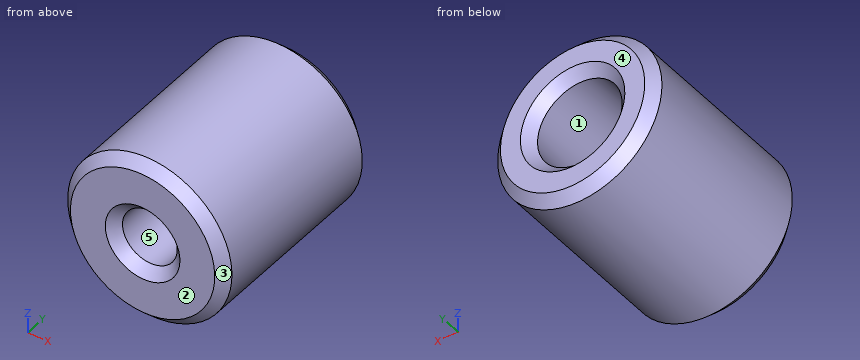
```python
from build123d import *

# Parameters (mm, degrees)
CHAMFER1_SIZE = 1


with BuildPart() as part:
    # Sketch1 → Revolve1 (revolve)
    with BuildSketch(Plane(origin=(0, 0, 0), x_dir=(0, 0, -1), z_dir=(1, 0, 0)), mode=Mode.PRIVATE) as revolve1_sk:
        Polygon((-4.25, 20), (-4.25, 12), (-2.75, 8), (-2.75, 0), (-8.25, 0), (-8.25, 20), align=None)
    revolve(revolve1_sk.sketch.rotate(Axis((0, 0, 0), (0, 1, 0)), 180), axis=Axis((0, 0, 0), (0, 1, 0)))

    # Chamfer1
    chamfer1_edges = [part.edges().sort_by_distance(p)[0] for p in [
        (0, 20, 8.25),
        (0, 0, 8.25),
        (0, 0, 2.75),
        (0, 20, 4.25),
    ]]
    chamfer(chamfer1_edges, length=CHAMFER1_SIZE)


solid = part.part
```
Read the model definition and answer for the solid it produces. Units are mm, in the model's axes. Face numbers are marked on the shaded views. A direction names the side the tool comes from. Give positions to 0.01 mm unless a question says otherwise; leave off trailing zeros. Order: outer loops, then holes, each group sorted by start corner. A loop starts at its lowest first (then second) coordinate and runs counter-clockwise, first axis right, second up. Notation, with made-up numbers: (-15, 55) -> (26, 55) arc R24 ccw to (26, 74) -> close; hole circle Ø8 at (41, 26). An arc over 180 degrees is marked (long way). Write item = value, one per line.
1. A cutting plane is placed at C-C, the plane y = 14.25. Write down the section's boundary in (x, z).
Numbers:
outline = circle Ø16.5 at (0, 0); hole circle Ø8.5 at (0, 0)
2. The mould has two halves that part along Y. Classify the marked faces 3, 4 and 5: +Y half, -Y half, draft (parallel to the pull), parting line (faces both ways), or undercut.
Numbers:
face_3 = -Y half
face_4 = +Y half
face_5 = draft
3. Straight lines are drawn through the part: line 1 along X through (y, z) = (17.75, 0); line 2 along X through (y, z) = (3.25, 0); line 3 along Z through (x, y) = (-1.5, 2.5). For each, find the intervals that lie inside material, in ascending order.
Numbers:
line_1 = -8.25 to -4.25, 4.25 to 8.25
line_2 = -8.25 to -2.75, 2.75 to 8.25
line_3 = -8.11 to -2.3, 2.3 to 8.11
4. For the marked faces 1 and 2, determine the directions among +Z, -Z, +X, -X, +Y, -Y from which every point of the face is accessible in a straight line to the end or side of a thin tool.
Numbers:
face_1 = +Y
face_2 = +Z, -Z, +X, -X, -Y
5. Given pin 1 (1.5 mm diameter, centred on x = -5, z = -6.5, fed in from +Y); pin 2 (9 mm diameter, centred on x = 0, z = 0, fed in from +Y), each flat-ended and moving along its own axis, determine where each tip first touches the part or whether it passes through.
Numbers:
pin_1 = 19.8
pin_2 = 19.25
6. A cutting plane is placed at B-B, the plane x = 0. Write down the section's boundary in (y, z), and give its area (3 significant figures).
Numbers:
outline = (0, -7.25) -> (1, -8.25) -> (19, -8.25) -> (20, -7.25) -> (20, -5.25) -> (19, -4.25) -> (12, -4.25) -> (8, -2.75) -> (1, -2.75) -> (0, -3.75) -> close; (0, 3.75) -> (1, 2.75) -> (8, 2.75) -> (12, 4.25) -> (19, 4.25) -> (20, 5.25) -> (20, 7.25) -> (19, 8.25) -> (1, 8.25) -> (0, 7.25) -> close
area = 186 mm²
7. A cutting plane is placed at A-A, the plane z = 0. Write down the section's boundary in (x, y), and give its area (3 significant figures).
Numbers:
outline = (-8.25, 1) -> (-7.25, 0) -> (-3.75, 0) -> (-2.75, 1) -> (-2.75, 8) -> (-4.25, 12) -> (-4.25, 19) -> (-5.25, 20) -> (-7.25, 20) -> (-8.25, 19) -> close; (2.75, 1) -> (3.75, 0) -> (7.25, 0) -> (8.25, 1) -> (8.25, 19) -> (7.25, 20) -> (5.25, 20) -> (4.25, 19) -> (4.25, 12) -> (2.75, 8) -> close
area = 186 mm²
8. A cutting plane is placed at D-D, the plane y = 7.25. Write down the section's boundary in (x, z), and give its area (3 significant figures).
Numbers:
outline = circle Ø16.5 at (0, 0); hole circle Ø5.5 at (0, 0)
area = 190 mm²
